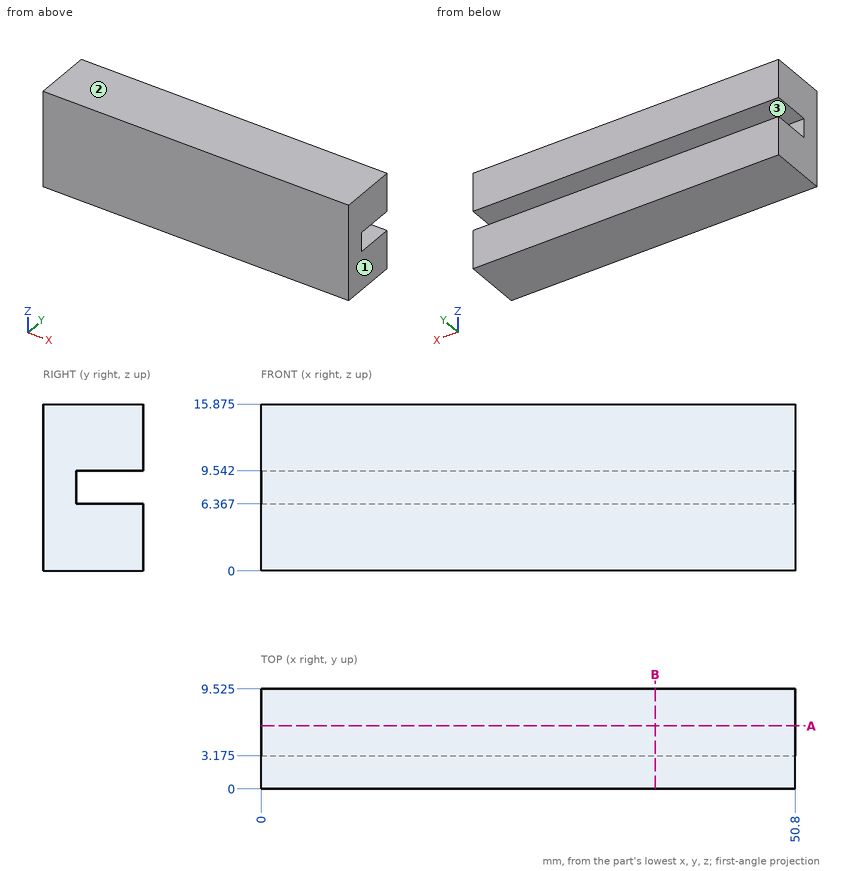
Study the drawing (mm; zero at the part's minimum x, y, z) and answer. Give positions to 0.01 mm unless a question says otherwise; leave off trailing zeros. Write each loop counter-clockwise with the first axis right and the second up, starting at its lowest first coordinate (ties: lowest second). Pieces come first, ordered by that corner, then holes.
(1) The part is cut by section A-A on y = 6. Write down the section's boundary in (x, z) (1 decimal).
Final values:
outline: (0, 0) - (50.8, 0) - (50.8, 6.4) - (0, 6.4) - close; (0, 9.5) - (50.8, 9.5) - (50.8, 15.9) - (0, 15.9) - close
(2) Straight lines are drawn through the part: line 1 (Z direction, x = 39, y = 5.75) (1 decimal); line 2 (Y direction, x = 4, z = 8) (3 decimals). For each, find the intervals that lie inside material, in ascending order.
Final values:
line 1: z = 0 to 6.4, 9.5 to 15.9
line 2: y = 0 to 3.175
(3) The mould has two halves that part along Z. Classify the marked faces 1, 2 and 3: pulls with the +Z half, pulls with the -Z half, needs draft (parallel to the pull), parting line crosses it, or undercut.
Final values:
face 1: needs draft
face 2: pulls with the +Z half
face 3: undercut
(4) The part is cut by section B-B on x = 37.5. Write down the section's boundary in (y, z) (1 decimal), plus the area to 3 significant figures.
Final values:
outline: (0, 0) - (9.5, 0) - (9.5, 6.4) - (3.2, 6.4) - (3.2, 9.5) - (9.5, 9.5) - (9.5, 15.9) - (0, 15.9) - close
area: 131 mm2
